The model under review builds one solid part; all positions refer to its coordinate system, in mm. A direction names the side the tool comes from. Coordinates: 2 decimals unless noted, no trailing zeros. Loops run counter-clockwise (first coordinate to the right, second up) from the corner with the lowest first, then second, coordinate; pieces in that order, holes last. Notation, with made-up numbers: (53, 78) - (91, 78) arc R27 ccw to (91, 95) - close; hole circle Ø2 at (16, -6.75). An arc over 180 degrees is marked (long way). Answer in a Markdown table with one row per item. Add a question column.
(1) We need section B-B on x = 22.5. Write out the cut boundary in (y, z), plus the area to 3 significant figures.
(2) We need section A-A on z = 0. Write out the cut boundary in (x, y), plus the area to 3 significant figures.
(3) Mouldability with a two-part tool opening along Y and no side actions: class faces 6 (the flat face through (13, 7, 10.16)), 7 (the cylindrical face through (12.88, 19.06, 87.82)), 8 (the flat face through (9.7, -10.16, -0.1)), 9 (the cylindrical face through (1.528, 102.852, 121.741)) as +Y half, -Y half, draft (parallel to the pull), parting line (faces both ways), or undercut.
(4) Machinability: for faces 1 (the flat face through (13, 101.6, 118)), 2 (the cylindrical face through (21.6, 42.4, 113.2)), 3 (the flat face through (13, -7, 10.16)), 4 (the cylindrical face through (3.8, 42.4, 113.2)), 5 (the cylindrical face through (15.447, -12.664, 0.121)), which of the approach directions +Z, -Z, +X, -X, +Y, -Y give a long, thin tool a straight path to every point of the face, cutting with its end or side? Answer none if there is none.
(5) For P1, Ø4, axis at x = 4, z = 73, coming from the +Y side; P2, Ø8, axis at x = 9, y = 5.5, coming from the -Z side; P3, Ø10, axis at x = 5, y = 53, coming from the +Z side, all flat-tipped, find the tip position at first contact; note any pin that passes through.
(6) We need section D-D on z = 48. Write out the cut boundary in (x, y).
(7) For line 1 along Y through (x, z) = (4, 38.5); line 2 along Z through (x, y) = (12.75, 60); line 3 along X through (y, z) = (32.5, 112), list the stretches that pass through material, from the lowest coordinate up.
from build123d import *

# Parameters (mm, degrees)
F1_DEPTH = 25.4
F2_R     = 12.69999
F3_R     = 5.08
F4_R     = 12.7
F6_D     = 5.5
F6_DEPTH = 5.588
F6_TIP   = 1.6523667023


# Not quite as in the source:
# - a fillet or chamfer is up to 0.001 mm smaller than in the source, because OpenCascade refuses the exact size


with BuildPart() as f1:
    # F0 (on Right) → F1 (new body)
    with BuildSketch(Plane.YZ):
        with BuildLine():
            Line((3.048, 10.16), (10.16, 10.16))
            Line((10.16, 10.16), (10.16, -10.16))
            Line((10.16, -10.16), (15.24, -10.16))
            Line((15.24, -10.16), (15.24, 91.44))
            Line((15.24, 91.44), (104.14, 91.44))
            Line((104.14, 91.44), (104.14, 123.19))
            Line((104.14, 123.19), (101.6, 123.19))
            Line((101.6, 123.19), (101.6, 116.84))
            Line((101.6, 116.84), (-15.24, 116.84))
            Line((-15.24, 116.84), (-15.24, -10.16))
            Line((-15.24, -10.16), (-10.16, -10.16))
            Line((-10.16, -10.16), (-10.16, 10.16))
            Line((-10.16, 10.16), (-3.048, 10.16))
            Line((-3.048, 10.16), (-3.048, 6.858))
            ThreePointArc((-3.048, 6.858), (-2.3040512242, 5.0619487758), (-0.508, 4.318))
            Line((-0.508, 4.318), (0.508, 4.318))
            ThreePointArc((0.508, 4.318), (2.3040512242, 5.0619487758), (3.048, 6.858))
            Line((3.048, 6.858), (3.048, 10.16))
        make_face()
    extrude(amount=F1_DEPTH)

    # F2 (radius 12.7 in the source; OpenCascade refuses exactly that, so slightly less here)
    f2_edges = [f1.edges().sort_by_distance(p)[0] for p in [
        (25.4, 43.18, 116.84),
        (0, 43.18, 116.84),
    ]]
    fillet(f2_edges, radius=F2_R)

    # F3
    f3_edges = [f1.edges().sort_by_distance(p)[0] for p in [
        (0, 102.87, 123.19),
        (25.4, 102.87, 123.19),
    ]]
    fillet(f3_edges, radius=F3_R)

    # F4
    f4_edges = [f1.edges().sort_by_distance(p)[0] for p in [
        (12.7, 15.24, 91.44),
    ]]
    fillet(f4_edges, radius=F4_R)

    # F6
    with Locations(Plane.XZ.offset(15.24)):
        with Locations((12.7, 0)):
            Hole(F6_D / 2, depth=F6_DEPTH)
            with Locations((0, 0, -(F6_DEPTH + F6_TIP / 2))):  # 118° drill point
                Cone(0, F6_D / 2, F6_TIP, mode=Mode.SUBTRACT)


solid = f1.part
Outcome:
| question | item | result |
|---|---|---|
| 1 | outline | (-15.24, -10.16) - (-10.16, -10.16) - (-10.16, 10.16) - (-3.05, 10.16) - (-3.05, 6.86) arc R2.54 ccw to (-0.51, 4.32) - (0.51, 4.32) arc R2.54 ccw to (3.05, 6.86) - (3.05, 10.16) - (10.16, 10.16) - (10.16, -10.16) - (15.24, -10.16) - (15.24, 78.74) arc R12.7 cw to (27.94, 91.44) - (104.14, 91.44) - (104.14, 122.7) - (101.6, 122.7) - (101.6, 112.22) - (-15.24, 112.22) - close |
| 1 | area | 5,260 mm² |
| 2 | outline | (0, -15.24) - (9.95, -15.24) - (9.95, -10.16) - (0, -10.16) - close; (0, 10.16) - (25.4, 10.16) - (25.4, 15.24) - (0, 15.24) - close; (15.45, -15.24) - (25.4, -15.24) - (25.4, -10.16) - (15.45, -10.16) - close |
| 2 | area | 230 mm² |
| 3 | face 6 | undercut |
| 3 | face 7 | +Y half |
| 3 | face 8 | undercut |
| 3 | face 9 | draft |
| 4 | face 1 | +Z, -Y |
| 4 | face 2 | +Z, +X, -Y |
| 4 | face 3 | -Z, +X, -X |
| 4 | face 4 | +Z, -X, -Y |
| 4 | face 5 | -Y |
| 5 | P1 | y = 15.24 |
| 5 | P2 | z = 4.52 |
| 5 | P3 | z = 116.55 |
| 6 | outline | (0, -15.24) - (25.4, -15.24) - (25.4, 15.24) - (0, 15.24) - close |
| 7 | line 1 | -15.24 to 15.24 |
| 7 | line 2 | 91.44 to 116.84 |
| 7 | line 3 | 2.72 to 22.68 |
